```python
from build123d import *

# Parameters (mm, degrees)
SKETCH2_W           = 92
SKETCH2_H           = 92
BOSS_EXTRUDE1_DEPTH = 38.2
SKETCH3_R           = 2.5
BOSS_EXTRUDE2_DEPTH = 10
SKETCH4_R           = 46
BOSS_EXTRUDE3_DEPTH = 10


with BuildPart() as part:
    # Sketch2 → Boss-Extrude1 (new body)
    with BuildSketch(Plane.XY):
        with Locations((46, 46)):
            Rectangle(SKETCH2_W, SKETCH2_H)
    extrude(amount=BOSS_EXTRUDE1_DEPTH)

    # Sketch3 → Boss-Extrude2 (add)
    with BuildSketch(Plane(origin=(0, 0, 0), x_dir=(-1, 0, 0), z_dir=(0, 0, -1))):
        with Locations((-4.98, 4.98)):
            Circle(SKETCH3_R)
        with Locations((-87.02, 4.98)):
            Circle(SKETCH3_R)
        with Locations((-87.02, 87.02)):
            Circle(SKETCH3_R)
        with Locations((-4.98, 87.02)):
            Circle(SKETCH3_R)
    extrude(amount=BOSS_EXTRUDE2_DEPTH)

    # Sketch4 → Boss-Extrude3 (add)
    with BuildSketch(Plane(origin=(0, 0, 0), x_dir=(-1, 0, 0), z_dir=(0, 0, -1))):
        with Locations((-46, 46)):
            Circle(SKETCH4_R)
    extrude(amount=BOSS_EXTRUDE3_DEPTH)


solid = part.part
```
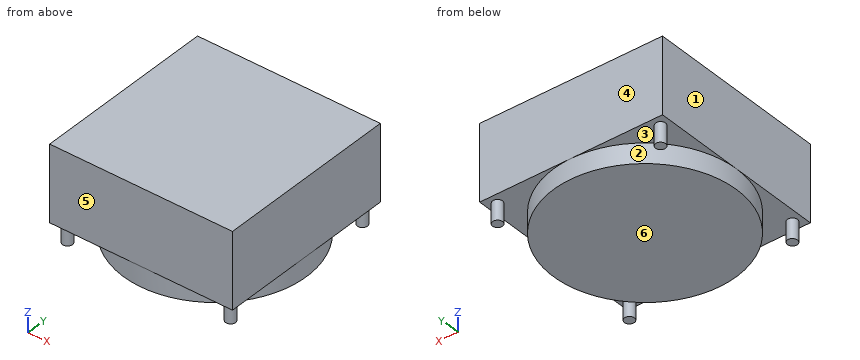
Check sheet for the modelled part. Datum: model origin and axes. Units: mm. Face numbers are marked on the shaded views. A direction names the side the tool comes from. Coordinates: 2 decimals unless noted, no trailing zeros. Order: outer loops, then holes, each group sorted by start corner. A loop starts at its lowest first (then second) coordinate and runs counter-clockwise, first axis right, second up. Notation, with made-up numbers: (-12, 57.5) -> (12, 57.5) arc R14 ccw to (12, 67.5) -> close; hole circle Ø5 at (-36.5, -24). An arc over 180 degrees is marked (long way). Write item = value, one per line. Start each with the question number.
1) Cross-section at C-C (y = 28). Enter the section's corners in (x, z), then the cut area to 3 significant figures.
2) Mould release check, pull along Y, two halves, no side actions. Record for the marked faces 3, 4, 5 and 6: +Y half, -Y half, draft (parallel to the pull), parting line (faces both ways), or undercut.
3) Access from +Z, -Z, +X, -X, +Y, -Y to the whole of each face (thin tool, end or side, straight path). Record for the marked faces 1 and 2.
4) Cross-section at D-D (x = 26.5). Enter the section's corners in (y, z).
5) Material ranges on L1, parallel to Y at x = 84, z = -4.5; L2, parallel to Y at x = 50, z = -0.5; L3, parallel to X at y = 74.5, z = -4.5, recorded low to high.
6) Cross-section at A-A (x = 87.02). Enter the section's corners in (y, z), then the cut area to 3 significant figures.
Ans:
q1.outline = (0, 0) -> (3.67, 0) -> (3.67, -10) -> (88.33, -10) -> (88.33, 0) -> (92, 0) -> (92, 38.2) -> (0, 38.2) -> close
q1.area = 4,360 mm²
q2.face_3 = undercut
q2.face_4 = +Y half
q2.face_5 = -Y half
q2.face_6 = draft
q3.face_1 = +Z, -Z, -X, +Y, -Y
q3.face_2 = -Z
q4.outline = (0, 0) -> (4.34, 0) -> (4.34, -10) -> (87.66, -10) -> (87.66, 0) -> (92, 0) -> (92, 38.2) -> (0, 38.2) -> close
q5.L1 = 20.08 to 71.92
q5.L2 = 0.17 to 91.83
q5.L3 = 9.89 to 82.11
q6.outline = (0, 0) -> (2.48, 0) -> (2.48, -10) -> (7.48, -10) -> (7.48, 0) -> (25.18, 0) -> (25.18, -10) -> (66.82, -10) -> (66.82, 0) -> (84.52, 0) -> (84.52, -10) -> (89.52, -10) -> (89.52, 0) -> (92, 0) -> (92, 38.2) -> (0, 38.2) -> close
q6.area = 4,030 mm²
